Read the model definition and answer for the solid it produces. Units are mm, in the model's axes. A direction names the side the tool comes from. Coordinates: 2 decimals unless noted, no trailing zeros. Write each loop counter-clockwise with the first axis right and the second up, starting at its lowest first coordinate (ties: lowest second). Pieces come first, ordered by that corner, then holes.
1) Find the intervals of material crossed by line 1 (Z direction, x = 1.55, y = -11.2); line 2 (Y direction, x = -4.5, z = 16.5); line 3 (X direction, y = -10, z = 50.5), in increasing order.
2) Each of these flat-tipped pins is pushed along its axis until it touches: pin 1 Ø2 at (y, z) = (-9.5, 16) entering from -X; pin 2 Ø20 at (x, z) = (-13.5, 61) entering from -Y. Where does it stop, or does it pass through?
3) Which of the six approach directions +Z, -Z, +X, -X, +Y, -Y give full straight-line access (tool end or side, diameter ignored) to faces 5 (the face through (-13.6, -2.7, 82)), 6 (the face through (0, -10, 42))?
4) The part is cut by section A-A (z = 22.5). Determine the outline of the cut face in (x, y), then the cut area to 3 significant figures.
5) Determine the mould class of faces 1 (the face through (1.48, -10.46, 48.92)), 2 (the face through (-13.6, -2.6, 0)), 3 (the face through (1.479, -11.408, 20.914)), 4 (the face through (-20, -3, 40)) for opening direction Z: +Z half, -Z half, draft (parallel to the pull), parting line (faces both ways), or undercut.
6) The part is cut by section D-D (x = -3). Determine the outline of the cut face in (y, z).
7) The part is cut by section C-C (z = 5). Determine the outline of the cut face in (x, y), then the cut area to 3 significant figures.
8) The part is cut by section B-B (y = -11.2). Determine the outline of the cut face in (x, z).
Autodesk Fusion 360 part; units mm, degrees
sketch "스케치1" plane through (0, 0, 0) normal (1, 0, 0) x (0, 1, 0)
  line L0 (0, 0) -> (-16, 0)
  line L1 (-16, 0) -> (-16, 82)
  line L2 (-16, 82) -> (0, 82)
  line L3 (0, 82) -> (0, 0)
  line L4 (0, 0) -> (-6, 0)
  line L5 (-6, 0) -> (-6, 82)
  line L6 (-6, 82) -> (0, 82)
  line L7 (0, 82) -> (0, 0)
  line L8 (-6, 0) -> (-11.2, 0)
  line L9 (-11.2, 0) -> (-11.2, 22.5)
  line L10 (-11.2, 22.5) -> (-6, 22.5)
  line L11 (-6, 22.5) -> (-6, 0)
  circle A0 centre (-11.2, 22.5) radius 1.6
  line L12 (-11.2, 22.5) -> (-11.2, 47.5)
  circle A1 centre (-11.2, 47.5) radius 1.6
  line L13 (0, 0) -> (-3, 0)
  line L14 (-3, 0) -> (-3, 82)
  line L15 (-3, 82) -> (0, 82)
  line L16 (0, 82) -> (0, 0)
  dimension "d1" = 16
  dimension "d2" = 82
  dimension "d3" = 6
  dimension "d4" = 82
  dimension "d5" = 5.2
  dimension "d6" = 22.5
  dimension "d7" = 3.2
  dimension "d8" = 25
  dimension "d9" = 3.2
  dimension "d14" = 3
  dimension "d15" = 82
extrude "돌출1" add sketch "스케치1" along normal blind 3 contours L0 L5 L8 L9 L10 L11 A0 | L0 L1 L2 L5 L9 L10 A0
extrude "돌출2" add sketch "스케치1" along normal blind 3 contours L0 L2 L3 L4 L6 L7 L13 L14 L15 L16 | L0 L2 L4 L5 L6 L11 L14
extrude "돌출3" add sketch "스케치1" against normal blind 40 contours L0 L2 L3 L4 L6 L7 L13 L14 L15 L16
Reported:
1. line 1: z = 0 to 20.9, 24.1 to 45.9, 49.1 to 82
1. line 2: y = -3 to 0
1. line 3: x = 0 to 3
2. pin 1: stops at x = 0
2. pin 2: stops at y = -3
3. face 5: +Z, +X, -X, +Y, -Y
3. face 6: +Z, -Z, -X, -Y
4. outline: (-40, -3) - (0, -3) - (0, -9.6) - (3, -9.6) - (3, 0) - (-40, 0) - close; (0, -16) - (3, -16) - (3, -12.8) - (0, -12.8) - close
4. area: 158 mm2
5. face 1: undercut
5. face 2: -Z half
5. face 3: undercut
5. face 4: draft
6. outline: (-3, 0) - (0, 0) - (0, 82) - (-3, 82) - close
7. outline: (-40, -3) - (0, -3) - (0, -16) - (3, -16) - (3, 0) - (-40, 0) - close
7. area: 168 mm2
8. outline: (0, 0) - (3, 0) - (3, 20.9) - (0, 20.9) - close; (0, 24.1) - (3, 24.1) - (3, 45.9) - (0, 45.9) - close; (0, 49.1) - (3, 49.1) - (3, 82) - (0, 82) - close
